Part model, mm, in its own coordinate system. Give positions to 0.01 mm unless a question says otherwise; leave off trailing zeros. Order: outer loops, then holes, each group sorted by start corner. A loop starts at its lowest first (then second) coordinate and runs counter-clockwise, first axis right, second up. Notation, with made-up numbers: M -24,57.5 L 22,57.5 A30 cw 22,87.5 Z; hole C 0.25,72.25 d10. An arc over 180 degrees is marked long. One line per question, with ' | ' between items.
```python
from build123d import *

# Parameters (mm, degrees)
SKETCH1_R           = 40
BOSS_EXTRUDE1_DEPTH = 90
SKETCH2_R           = 35
CUT_EXTRUDE1_DEPTH  = 85
FILLET1_R           = 2
FILLET2_R           = 5


with BuildPart() as part:
    # Sketch1 → Boss-Extrude1 (new body)
    with BuildSketch(Plane(origin=(0, 0, 0), x_dir=(1, 0, 0), z_dir=(0, 1, 0))):
        with Locations(Location((0, 0, 0), (0, 0, 90))):
            Circle(SKETCH1_R)
    extrude(amount=BOSS_EXTRUDE1_DEPTH)

    # Sketch2 → Cut-Extrude1 (cut)
    with BuildSketch(Plane(origin=(0, 90, 0), x_dir=(1, 0, 0), z_dir=(0, 1, 0))):
        with Locations(Location((0, 0, 0), (0, 0, 270))):
            Circle(SKETCH2_R)
    extrude(amount=-CUT_EXTRUDE1_DEPTH, mode=Mode.SUBTRACT)

    # Fillet1
    fillet1_edges = [part.edges().sort_by_distance(p)[0] for p in [
        (0, 90, 40),
        (0, 90, -35),
    ]]
    fillet(fillet1_edges, radius=FILLET1_R)

    # Fillet2
    fillet2_edges = [part.edges().sort_by_distance(p)[0] for p in [
        (0, 0, 40),
        (0, 5, -35),
    ]]
    fillet(fillet2_edges, radius=FILLET2_R)


solid = part.part
```
1. Drop flat-ended pins along their axis: pin 1 (2 mm diameter, centred on y = 31.5, z = 10, fed in from +X); pin 2 (5 mm diameter, centred on y = 16, z = 18, fed in from +X); pin 3 (2 mm diameter, centred on x = 21.5, z = 2.5, fed in from +Y). Give the stop position or say it passes through.
Worked out:
pin 1: stops at x = 38.97 | pin 2: stops at x = 36.87 | pin 3: stops at y = 5
2. Slice it at B-B on z = 0. Give the cut face in (x, y).
Worked out:
outline: M -40,5 A5 ccw -35,0 L 35,0 A5 ccw 40,5 L 40,88 A2 ccw 38,90 L 37,90 A2 ccw 35,88 L 35,10 A5 cw 30,5 L -30,5 A5 cw -35,10 L -35,88 A2 ccw -37,90 L -38,90 A2 ccw -40,88 Z
3. Probe L1, parallel to X at y = 37.5, z = 0; L2, parallel to Y at x = -1, z = -15.5; L3, parallel to X at y = 75.5, z = 22. List the from-to ranges inside material, lowest first. Write a range as from..to.
Worked out:
L1: x = -40..-35, 35..40 | L2: y = 0..5 | L3: x = -33.41..-27.22, 27.22..33.41
4. Slice it at A-A on x = 0. Give the cut face in (y, z), then the cut area to 3 significant figures.
Worked out:
outline: M 0,-35 A5 ccw 5,-40 L 88,-40 A2 ccw 90,-38 L 90,-37 A2 ccw 88,-35 L 10,-35 A5 cw 5,-30 L 5,30 A5 cw 10,35 L 88,35 A2 ccw 90,37 L 90,38 A2 ccw 88,40 L 5,40 A5 ccw 0,35 Z | area: 1,250 mm2
5. Slice it at C-C on y = 40. Give the cut face in (x, z).
Worked out:
outline: C 0,0 d80; hole C 0,0 d70
6. Mould opens along X. For faces 1 (the flat face through (0, 5, 0)), 2 (the cylindrical face through (-21, 50, -28)), 3 (the cylindrical face through (39.05, 45.92, 8.67)), 4 (the flat face through (0, 0, 0)) say: released by +X, released by -X, zero draft, split by the parting line, or undercut.
Worked out:
face 1: undercut | face 2: undercut | face 3: split by the parting line | face 4: zero draft
